from build123d import *

# Parameters (mm, degrees)
BOSS_EXTRUDE1_DEPTH = 49.022
CHAMFER4_SIZE       = 3.175
CHAMFER5_SIZE       = 3.175
CHAMFER6_SIZE       = 3.175
SKETCH4_R           = 2.178410544
CUT_EXTRUDE1_DEPTH  = 5.08
CHAMFER7_SIZE       = 1.27
CHAMFER8_SIZE       = 1.27
CHAMFER9_SIZE       = 1.27


with BuildPart() as part:
    # Sketch1 → Boss-Extrude1 (new body)
    with BuildSketch(Plane(origin=(0, 0, 0), x_dir=(0, 0, -1), z_dir=(1, 0, 0))):
        Polygon((19.343076923, 8.689730769), (27.832538462, 8.689730769), (27.832538462, -14.453576923), (-25.253461538, -14.453576923), (-25.253461538, -3.385038462), (-11.820769231, -3.385038462), (-11.820769231, 22.122423077), (19.343076923, 22.122423077), align=None)
    extrude(amount=BOSS_EXTRUDE1_DEPTH)

    # Chamfer4
    chamfer4_edges = [part.edges().sort_by_distance(p)[0] for p in [
        (0, 22.122423077, -3.761153846),
    ]]
    chamfer(chamfer4_edges, length=CHAMFER4_SIZE)

    # Chamfer5
    chamfer5_edges = [part.edges().sort_by_distance(p)[0] for p in [
        (49.022, 22.122423077, -3.761153846),
    ]]
    chamfer(chamfer5_edges, length=CHAMFER5_SIZE)

    # Chamfer6
    chamfer6_edges = [part.edges().sort_by_distance(p)[0] for p in [
        (0, -2.881923077, -27.832538462),
        (0, -8.919307692, 25.253461538),
        (49.022, -2.881923077, -27.832538462),
        (49.022, -8.919307692, 25.253461538),
    ]]
    chamfer(chamfer6_edges, length=CHAMFER6_SIZE)

    # Sketch4 → Cut-Extrude1 (cut)
    with BuildSketch(Plane(origin=(0, -3.385038462, 0), x_dir=(1, 0, 0), z_dir=(0, 1, 0))):
        with Locations(Location((24.66531327, -18.90809717, 0), (0, 0, 270))):
            Circle(SKETCH4_R)
        with Locations(Location((37.36531327, -18.90809717, 0), (0, 0, 270))):
            Circle(SKETCH4_R)
        with Locations(Location((11.96531327, -18.90809717, 0), (0, 0, 270))):
            Circle(SKETCH4_R)
    extrude(amount=-CUT_EXTRUDE1_DEPTH, mode=Mode.SUBTRACT)

    # Chamfer7
    chamfer7_edges = [part.edges().sort_by_distance(p)[0] for p in [
        (49.022, 8.689730769, -22.000307692),
        (0, 8.689730769, -22.000307692),
        (24.511, 8.689730769, -27.832538462),
        (1.5875, 8.689730769, -26.245038462),
        (47.4345, 8.689730769, -26.245038462),
    ]]
    chamfer(chamfer7_edges, length=CHAMFER7_SIZE)

    # Chamfer8
    chamfer8_edges = [part.edges().sort_by_distance(p)[0] for p in [
        (0, -3.385038462, 16.949615385),
        (49.022, -3.385038462, 16.949615385),
        (24.511, -3.385038462, 25.253461538),
        (1.5875, -3.385038462, 23.665961538),
        (47.4345, -3.385038462, 23.665961538),
    ]]
    chamfer(chamfer8_edges, length=CHAMFER8_SIZE)

    # Chamfer9
    chamfer9_edges = [part.edges().sort_by_distance(p)[0] for p in [
        (1.5875, 20.534923077, 11.820769231),
        (1.5875, 20.534923077, -19.343076923),
        (24.511, 22.122423077, 11.820769231),
        (47.4345, 20.534923077, 11.820769231),
        (24.511, 22.122423077, -19.343076923),
        (47.4345, 20.534923077, -19.343076923),
    ]]
    chamfer(chamfer9_edges, length=CHAMFER9_SIZE)


solid = part.part
The listing builds one solid part. Answer for the finished solid, in the listing's coordinates (mm). A direction names the side the tool comes from. Coordinates: 2 decimals unless noted, no trailing zeros. Loops run counter-clockwise (first coordinate to the right, second up) from the corner with the lowest first, then second, coordinate; pieces in that order, holes last. Notation, with made-up numbers: (-0.75, -5) -> (17.25, -5) arc R8 cw to (17.25, 9) -> close; hole circle Ø7 at (28, 68). An arc over 180 degrees is marked (long way). Write item = value, one per line. Start each with the question number.
1) A cutting plane is placed at B-B (y = 3). Give the vertices of the cut face in (x, z) (3 decimals).
2) A cutting plane is placed at D-D (x = 36.5). Give the vertices of the cut face in (y, z), then the cut area to 3 significant figures.
3) A cutting plane is placed at C-C (z = -22.5). Give the vertices of the cut face in (x, y).
4) Given pin 1 Ø5 at (x, z) = (11.5, 19) entering from +Y; pin 2 Ø8 at (x, z) = (16.5, -24.5) entering from +Y; pin 3 Ø4 at (x, y) = (23.5, 14) entering from -Z, each flat-ended and moving along its own axis, determine where each tip first touches the part or whether it passes through.
5) The mould has two halves that part along X. Classify faces 1 (the face through (24.212, 21.479, -18.717)), 2 (the face through (1.622, 19.659, -18.717)), 3 (the face through (37, -8.465, 19)): released by +X, released by -X, zero draft, split by the parting line, or undercut.
6) A tool of negligible diameter and unlimited length cuts with its end or side. For faces 4 (the face through (24, -3, -27.833)), 5 (the face through (25, -8.465, 19)), 6 (the face through (48.38, 8.06, -21.96)), 7 (the face through (48.378, -4.011, 17.021)), from which of +Z, -Z, +X, -X, +Y, -Y can it reach the whole face along a straight path? Write none if from no direction.
7) Straight lines are drawn through the part: line 1 (Y direction, x = 23, z = 21.5); line 2 (Z direction, x = 3, y = 10); line 3 (Z direction, x = 25.5, y = 3.5). For each, find the intervals that lie inside material, in ascending order. Write a range as from..to.
8) A cutting plane is placed at A-A (x = 16). Give the vertices of the cut face in (y, z).
Responses:
q1.outline = (0, -24.658) -> (3.175, -27.833) -> (45.847, -27.833) -> (49.022, -24.658) -> (49.022, 11.821) -> (0, 11.821) -> close
q2.outline = (-14.45, -27.83) -> (7.42, -27.83) -> (8.69, -26.56) -> (8.69, -19.34) -> (20.85, -19.34) -> (22.12, -18.07) -> (22.12, 10.55) -> (20.85, 11.82) -> (-3.39, 11.82) -> (-3.39, 16.91) -> (-8.47, 16.91) -> (-8.47, 20.91) -> (-3.39, 20.91) -> (-3.39, 23.98) -> (-4.66, 25.25) -> (-14.45, 25.25) -> close
q2.area = 1,460 mm²
q3.outline = (0, -14.45) -> (49.02, -14.45) -> (49.02, 7.42) -> (47.75, 8.69) -> (1.27, 8.69) -> (0, 7.42) -> close
q4.pin_1 = -3.39
q4.pin_2 = 8.69
q4.pin_3 = -19.34
q5.face_1 = zero draft
q5.face_2 = released by -X
q5.face_3 = undercut
q6.face_4 = -Z, +X, -X, +Y, -Y
q6.face_5 = +Y
q6.face_6 = -Z, +X, +Y
q6.face_7 = +Z, +X, +Y
q7.line_1 = -14.45..-3.39
q7.line_2 = -19.34..11.82
q7.line_3 = -27.83..11.82
q8.outline = (-14.45, -27.83) -> (7.42, -27.83) -> (8.69, -26.56) -> (8.69, -19.34) -> (20.85, -19.34) -> (22.12, -18.07) -> (22.12, 10.55) -> (20.85, 11.82) -> (-3.39, 11.82) -> (-3.39, 23.98) -> (-4.66, 25.25) -> (-14.45, 25.25) -> close
